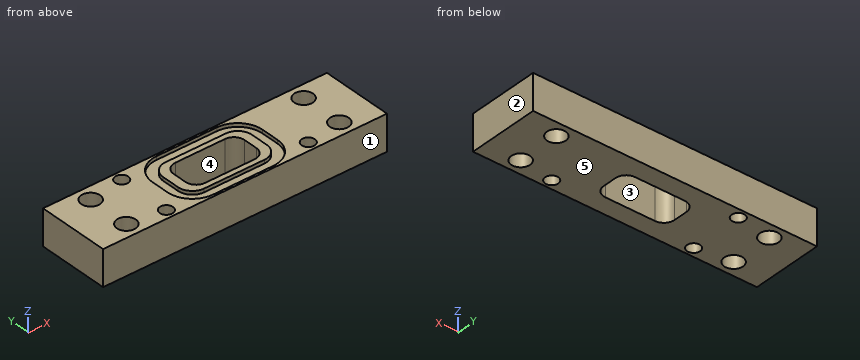
from build123d import *

# Parameters (mm, degrees)
SKIZZE1_W                        = 80
SKIZZE1_H                        = 20.2
SKIZZE1_R                        = 2.65
SKIZZE1_W_2                      = 20
SKIZZE1_H_2                      = 10
AUFSATZ_LINEAR_AUSTRAGEN1_DEPTH  = 10
VERRUNDUNG1_R                    = 3
F_3_7_3_7_DURCHMESSER_BOHRUNG1_D = 3.7
SCHNITT_LINEAR_AUSTRAGEN1_DEPTH  = 1


with BuildPart() as part:
    # Skizze1 → Aufsatz-Linear austragen1 (new body)
    with BuildSketch(Plane.XY):
        with Locations((40, 10.1)):
            Rectangle(SKIZZE1_W, SKIZZE1_H)
        with Locations((10, 16.1)):
            Circle(SKIZZE1_R, mode=Mode.SUBTRACT)
        with Locations((10, 4.1)):
            Circle(SKIZZE1_R, mode=Mode.SUBTRACT)
        with Locations((70, 16.1)):
            Circle(SKIZZE1_R, mode=Mode.SUBTRACT)
        with Locations((70, 4.1)):
            Circle(SKIZZE1_R, mode=Mode.SUBTRACT)
        with Locations((40, 10.1)):
            Rectangle(SKIZZE1_W_2, SKIZZE1_H_2, mode=Mode.SUBTRACT)
    extrude(amount=AUFSATZ_LINEAR_AUSTRAGEN1_DEPTH)

    # Verrundung1
    verrundung1_edges = [part.edges().sort_by_distance(p)[0] for p in [
        (50, 5.1, 5),
        (50, 15.1, 5),
        (30, 15.1, 5),
        (30, 5.1, 5),
    ]]
    fillet(verrundung1_edges, radius=VERRUNDUNG1_R)

    # Ø3.7 (3.7) Durchmesser Bohrung1 (through all)
    with Locations(Plane.XY.offset(10)):
        with Locations((20, 17.6), (20, 2.6), (60, 2.6)):
            Hole(F_3_7_3_7_DURCHMESSER_BOHRUNG1_D / 2)

    # Skizze7 → Schnitt-Linear austragen1 (cut)
    with BuildSketch(Plane.XY.offset(10)):
        with BuildLine():
            Line((24.5, 12.6), (24.5, 7.6))
            ThreePointArc((24.5, 7.6), (26.550252532, 2.650252532), (31.5, 0.6))
            Line((31.5, 0.6), (48.5, 0.6))
            ThreePointArc((48.5, 0.6), (53.449747468, 2.650252532), (55.5, 7.6))
            Line((55.5, 7.6), (55.5, 12.6))
            ThreePointArc((55.5, 12.6), (53.449747468, 17.549747468), (48.5, 19.6))
            Line((48.5, 19.6), (31.5, 19.6))
            ThreePointArc((31.5, 19.6), (26.550252532, 17.549747468), (24.5, 12.6))
        make_face()
        with BuildLine():
            Line((31.5, 16.6), (48.5, 16.6))
            ThreePointArc((48.5, 16.6), (51.328427125, 15.428427125), (52.5, 12.6))
            Line((52.5, 12.6), (52.5, 7.6))
            ThreePointArc((52.5, 7.6), (51.328427125, 4.771572875), (48.5, 3.6))
            Line((48.5, 3.6), (31.5, 3.6))
            ThreePointArc((31.5, 3.6), (28.671572875, 4.771572875), (27.5, 7.6))
            Line((27.5, 7.6), (27.5, 12.6))
            ThreePointArc((27.5, 12.6), (28.671572875, 15.428427125), (31.5, 16.6))
        make_face(mode=Mode.SUBTRACT)
    extrude(amount=-SCHNITT_LINEAR_AUSTRAGEN1_DEPTH, mode=Mode.SUBTRACT)


solid = part.part
Model file for the job. Use its own axes, mm. Face numbers are marked on the shaded views. A direction names the side the tool comes from. Round coordinates to 2 decimals unless told otherwise and drop trailing zeros. Order: outer loops, then holes, each group sorted by start corner. A loop starts at its lowest first (then second) coordinate and runs counter-clockwise, first axis right, second up. Notation, with made-up numbers: M 42,60.25 L 60,60.25 A17 ccw 60,91.25 Z; hole C 21.5,-35 d4. An arc over 180 degrees is marked long. Write each question's results on one line, items separated by ' | '. Start each with the question number.
(1) Saw through at C-C, the plane z = 5. State how many separate pieces and enclosed holes the cut face has, then the cut area to 3 significant figures.
(2) Saw through at A-A, the plane x = 70. Give the cut face in (y, z).
(3) Drop flat-ended pins along their axis: pin 1 (2 mm diameter, centred on x = 32.5, y = 2.5, fed in from +Z); pin 2 (5 mm diameter, centred on x = 70, y = 16.1, fed in from -Z). Give the stop position or say it passes through.
(4) Saw through at D-D, the plane x = 40. Give the cut face in (y, z).
(5) Probe probe 1 along Y at (x, z) = (70, 3); probe 2 along Y at (x, z) = (60, 5.75); probe 3 along Y at (x, z) = (19.5, 4.25). List the from-to ranges inside material, lowest first. Write a range as from..to.
(6) Saw through at B-B, the plane y = 9. Give the cut face in (x, z).
(7) Two-plate mould, pull along X, no slides. Class the marked faces 1, 2 and 3: pulls with the +X half, pulls with the -X half, needs draft (parallel to the pull), parting line crosses it, or undercut.
(8) Which spindle directions (+Z, -Z, +X, -X, +Y, -Y) get a long thin tool onto all of the face, cutting with end or side? Do the marked faces 4 and 5. Say none if no direction does.
Established:
1) separate pieces: 1 | enclosed holes: 8 | area: 1,300 mm^2
2) outline: M 0,0 L 1.45,0 L 1.45,10 L 0,10 Z; M 6.75,0 L 13.45,0 L 13.45,10 L 6.75,10 Z; M 18.75,0 L 20.2,0 L 20.2,10 L 18.75,10 Z
3) pin 1: stops at z = 9 | pin 2: passes through
4) outline: M 0,0 L 5.1,0 L 5.1,10 L 3.6,10 L 3.6,9 L 0.6,9 L 0.6,10 L 0,10 Z; M 15.1,0 L 20.2,0 L 20.2,10 L 19.6,10 L 19.6,9 L 16.6,9 L 16.6,10 L 15.1,10 Z
5) probe 1: y = 0..1.45, 6.75..13.45, 18.75..20.2 | probe 2: y = 0..0.75, 4.45..20.2 | probe 3: y = 0..0.82, 4.38..15.82, 19.38..20.2
6) outline: M 0,0 L 30,0 L 30,10 L 27.5,10 L 27.5,9 L 24.5,9 L 24.5,10 L 0,10 Z; M 50,0 L 80,0 L 80,10 L 55.5,10 L 55.5,9 L 52.5,9 L 52.5,10 L 50,10 Z
7) face 1: needs draft | face 2: pulls with the +X half | face 3: undercut
8) face 4: +Z, -Z | face 5: -Z, +X, -X, +Y, -Y
